The listing builds one solid part. Answer for the finished solid, in the listing's coordinates (mm). A direction names the side the tool comes from. Coordinates: 2 decimals unless noted, no trailing zeros. Order: outer loops, then holes, each group sorted by start corner. A loop starts at its lowest first (then second) coordinate and runs counter-clockwise, first axis right, second up. Notation, with made-up numbers: (-34.5, 14) -> (20.5, 14) arc R23 ccw to (20.5, 26) -> close; hole circle Ø10 at (32, 3). An arc over 180 degrees is marked (long way). Write item = value, one per line.
from build123d import *

# Parameters (mm, degrees)
SKETCH1_W           = 120
SKETCH1_H           = 120
BOSS_EXTRUDE1_DEPTH = 17
SHELL1_T            = -3
SKETCH2_W           = 124
SKETCH2_H           = 124
SKETCH2_W_2         = 120
SKETCH2_H_2         = 120
BOSS_EXTRUDE2_DEPTH = 5
SKETCH4_R           = 4.02
BOSS_EXTRUDE3_DEPTH = 14
SKETCH3_R           = 4.02
CUT_EXTRUDE1_DEPTH  = 3
FILLET1_R           = 10
SKETCH9_R           = 9.39878502
SKETCH9_R_2         = 4.690586007
SKETCH9_W           = 4.6868
SKETCH9_H           = 21.8714
BOSS_EXTRUDE7_DEPTH = 1


with BuildPart() as part:
    # Sketch1 → Boss-Extrude1 (new body)
    with BuildSketch(Plane(origin=(0, 0, 0), x_dir=(1, 0, 0), z_dir=(0, 1, 0))):
        Rectangle(SKETCH1_W, SKETCH1_H)
    extrude(amount=BOSS_EXTRUDE1_DEPTH)

    # Shell1
    shell1_openings = [part.faces().sort_by_distance(p)[0] for p in [
        (0, 0, 0),
    ]]
    offset(amount=SHELL1_T, openings=shell1_openings, kind=Kind.INTERSECTION)

    # Sketch2 → Boss-Extrude2 (add)
    with BuildSketch(Plane.XZ):
        Rectangle(SKETCH2_W, SKETCH2_H)
        Rectangle(SKETCH2_W_2, SKETCH2_H_2, mode=Mode.SUBTRACT)
    extrude(amount=-BOSS_EXTRUDE2_DEPTH)

    # Sketch4 → Boss-Extrude3 (add)
    # profile 1 of 4: a face of its own
    with BuildSketch(Plane.XZ.offset(-14)):
        with BuildLine():
            Line((-57, 42.98), (-57, 57))
            Line((-57, 57), (-42.98, 57))
            ThreePointArc((-42.98, 57), (-44.394213562, 56.414213562), (-44.98, 55))
            Line((-44.98, 55), (-44.98, 52))
            ThreePointArc((-44.98, 52), (-47.036110396, 47.036110396), (-52, 44.98))
            Line((-52, 44.98), (-55, 44.98))
            ThreePointArc((-55, 44.98), (-56.414213562, 44.394213562), (-57, 42.98))
        make_face()
        with Locations(Location((-52, 52, 0), (0, 0, 270))):
            Circle(SKETCH4_R, mode=Mode.SUBTRACT)
    # profile 2 of 4: a face of its own
    with BuildSketch(Plane.XZ.offset(-14)):
        with BuildLine():
            Line((57, 42.98), (57, 57))
            Line((57, 57), (42.98, 57))
            ThreePointArc((42.98, 57), (44.394213562, 56.414213562), (44.98, 55))
            Line((44.98, 55), (44.98, 52))
            ThreePointArc((44.98, 52), (47.036110396, 47.036110396), (52, 44.98))
            Line((52, 44.98), (55, 44.98))
            ThreePointArc((55, 44.98), (56.414213562, 44.394213562), (57, 42.98))
        make_face()
        with Locations(Location((52, 52, 0), (0, 0, 90))):
            Circle(SKETCH4_R, mode=Mode.SUBTRACT)
    # profile 3 of 4: a face of its own
    with BuildSketch(Plane.XZ.offset(-14)):
        with BuildLine():
            Line((55, -44.98), (52, -44.98))
            ThreePointArc((52, -44.98), (47.036110396, -47.036110396), (44.98, -52))
            Line((44.98, -52), (44.98, -55))
            ThreePointArc((44.98, -55), (44.394213562, -56.414213562), (42.98, -57))
            Line((42.98, -57), (57, -57))
            Line((57, -57), (57, -42.98))
            ThreePointArc((57, -42.98), (56.414213562, -44.394213562), (55, -44.98))
        make_face()
        with Locations(Location((52, -52, 0), (0, 0, 270))):
            Circle(SKETCH4_R, mode=Mode.SUBTRACT)
    # profile 4 of 4: a face of its own
    with BuildSketch(Plane.XZ.offset(-14)):
        with BuildLine():
            Line((-57, -42.98), (-57, -57))
            Line((-57, -57), (-42.98, -57))
            ThreePointArc((-42.98, -57), (-44.394213562, -56.414213562), (-44.98, -55))
            Line((-44.98, -55), (-44.98, -52))
            ThreePointArc((-44.98, -52), (-47.036110396, -47.036110396), (-52, -44.98))
            Line((-52, -44.98), (-55, -44.98))
            ThreePointArc((-55, -44.98), (-56.414213562, -44.394213562), (-57, -42.98))
        make_face()
        with Locations(Location((-52, -52, 0), (0, 0, 90))):
            Circle(SKETCH4_R, mode=Mode.SUBTRACT)
    extrude(amount=BOSS_EXTRUDE3_DEPTH)

    # Sketch3 → Cut-Extrude1 (cut)
    with BuildSketch(Plane(origin=(0, 17, 0), x_dir=(1, 0, 0), z_dir=(0, 1, 0))):
        with Locations(Location((-52, 52, 0), (0, 0, 270))):
            Circle(SKETCH3_R)
        with Locations(Location((52, 52, 0), (0, 0, 90))):
            Circle(SKETCH3_R)
        with Locations(Location((52, -52, 0), (0, 0, 270))):
            Circle(SKETCH3_R)
        with Locations(Location((-52, -52, 0), (0, 0, 90))):
            Circle(SKETCH3_R)
    extrude(amount=-CUT_EXTRUDE1_DEPTH, mode=Mode.SUBTRACT)

    # Fillet1
    fillet1_edges = [part.edges().sort_by_distance(p)[0] for p in [
        (62, 2.5, -62),
        (-62, 2.5, -62),
        (-62, 2.5, 62),
        (62, 2.5, 62),
        (60, 11, 60),
        (-60, 11, 60),
        (-60, 11, -60),
        (60, 11, -60),
    ]]
    fillet(fillet1_edges, radius=FILLET1_R)

    # Sketch9 → Boss-Extrude7 (add)
    # profile 1 of 8: a face of its own
    with BuildSketch(Plane(origin=(0, 17, 0), x_dir=(1, 0, 0), z_dir=(0, 1, 0))):
        with Locations(Location((0, 12.032739488, 0), (0, 0, 270))):
            Circle(SKETCH9_R)
        with Locations(Location((0, 12.032739488, 0), (0, 0, 270))):
            Circle(SKETCH9_R_2, mode=Mode.SUBTRACT)
    # profile 2 of 8: a face of its own
    with BuildSketch(Plane(origin=(0, 17, 0), x_dir=(1, 0, 0), z_dir=(0, 1, 0))):
        with BuildLine():
            Line((-13.44305, 20.375947386), (-17.50480026, 22.896805886))
            ThreePointArc((-17.50480026, 22.896805886), (0.002640651, 32.634825883), (17.507584665, 22.892318209))
            Line((17.507584665, 22.892318209), (13.445188322, 20.372501014))
            ThreePointArc((13.445188322, 20.372501014), (0.002027924, 27.854392601), (-13.44305, 20.375947386))
        make_face()
    # profile 3 of 8: a face of its own
    with BuildSketch(Plane(origin=(0, 17, 0), x_dir=(1, 0, 0), z_dir=(0, 1, 0))):
        with BuildLine():
            Line((-40.2286, -27.927144715), (-40.2286, 3.597555285))
            ThreePointArc((-40.2286, 3.597555285), (-37.592561031, 9.961516315), (-31.2286, 12.597555285))
            Line((-31.2286, 12.597555285), (-14.988446655, 12.597555285))
            Line((-14.988446655, 12.597555285), (-14.988446655, 7.597555285))
            Line((-14.988446655, 7.597555285), (-31.2286, 7.597555285))
            ThreePointArc((-31.2286, 7.597555285), (-34.057027125, 6.42598241), (-35.2286, 3.597555285))
            Line((-35.2286, 3.597555285), (-35.2286, -27.927144715))
            ThreePointArc((-35.2286, -27.927144715), (-34.057027125, -30.75557184), (-31.2286, -31.927144715))
            Line((-31.2286, -31.927144715), (31.2286, -31.927144715))
            ThreePointArc((31.2286, -31.927144715), (34.057027125, -30.75557184), (35.2286, -27.927144715))
            Line((35.2286, -27.927144715), (35.2286, 3.597555285))
            ThreePointArc((35.2286, 3.597555285), (34.057027125, 6.42598241), (31.2286, 7.597555285))
            Line((31.2286, 7.597555285), (14.988446655, 7.597555285))
            Line((14.988446655, 7.597555285), (14.988446655, 12.597555285))
            Line((14.988446655, 12.597555285), (31.2286, 12.597555285))
            ThreePointArc((31.2286, 12.597555285), (37.592561031, 9.961516315), (40.2286, 3.597555285))
            Line((40.2286, 3.597555285), (40.2286, -27.927144715))
            ThreePointArc((40.2286, -27.927144715), (37.592561031, -34.291105746), (31.2286, -36.927144715))
            Line((31.2286, -36.927144715), (-31.2286, -36.927144715))
            ThreePointArc((-31.2286, -36.927144715), (-37.592561031, -34.291105746), (-40.2286, -27.927144715))
        make_face()
    # profile 4 of 8: a face of its own
    with BuildSketch(Plane(origin=(0, 17, 0), x_dir=(1, 0, 0), z_dir=(0, 1, 0))):
        with BuildLine():
            Line((-22.967626314, 26.287219035), (-26.8861, 28.719155285))
            ThreePointArc((-26.8861, 28.719155285), (0.004055848, 43.676045714), (26.890376645, 28.712262541))
            Line((26.890376645, 28.712262541), (22.971279665, 26.281330863))
            ThreePointArc((22.971279665, 26.281330863), (0.003464735, 39.064240253), (-22.967626314, 26.287219035))
        make_face()
    # profile 5 of 8: a face of its own
    with BuildSketch(Plane(origin=(0, 17, 0), x_dir=(1, 0, 0), z_dir=(0, 1, 0))):
        with BuildLine():
            Line((-27.8078, -24.037744715), (-27.8077, -2.166344715))
            Line((-27.8077, -2.166344715), (-19.6684, -2.322544715))
            ThreePointArc((-19.6684, -2.322544715), (-14.083780395, -7.46632893), (-16.7627, -14.570544715))
            Line((-16.7627, -14.570544715), (-13.694775607, -23.959644715))
            Line((-13.694775607, -23.959644715), (-18.653, -23.959644715))
            Line((-18.653, -23.959644715), (-21.3088, -15.757844715))
            Line((-21.3088, -15.757844715), (-23.121, -15.757844715))
            Line((-23.121, -15.757844715), (-23.121, -24.037744715))
            Line((-23.121, -24.037744715), (-27.8078, -24.037744715))
        make_face()
        with BuildLine():
            Line((-23.1211, -6.853044715), (-23.1211, -11.071144715))
            Line((-23.1211, -11.071144715), (-20.688080887, -11.071144715))
            ThreePointArc((-20.688080887, -11.071144715), (-18.579030887, -8.962094715), (-20.688080887, -6.853044715))
            Line((-20.688080887, -6.853044715), (-23.1211, -6.853044715))
        make_face(mode=Mode.SUBTRACT)
    # profile 6 of 8: a face of its own
    with BuildSketch(Plane(origin=(0, 17, 0), x_dir=(1, 0, 0), z_dir=(0, 1, 0))):
        Polygon((-9.5295, -2.166244715), (-9.5295, -24.037744715), (-4.8428, -24.037744715), (-4.8428, -15.289144715), (-0.781, -15.289144715), (-0.781, -10.602344715), (-4.8428, -10.602344715), (-4.8428, -6.853044715), (1.25, -6.853044715), (1.25, -2.166244715), align=None)
    # profile 7 of 8: a face of its own
    with BuildSketch(Plane(origin=(0, 17, 0), x_dir=(1, 0, 0), z_dir=(0, 1, 0))):
        with Locations((7.4989, -13.102044715)):
            Rectangle(SKETCH9_W, SKETCH9_H)
    # profile 8 of 8: a face of its own
    with BuildSketch(Plane(origin=(0, 17, 0), x_dir=(1, 0, 0), z_dir=(0, 1, 0))):
        with BuildLine():
            Line((13.904, -2.135144715), (13.904, -24.068944715))
            Line((13.904, -24.068944715), (22.62153415, -24.068944715))
            ThreePointArc((22.62153415, -24.068944715), (29.187351473, -13.102044715), (22.62153415, -2.135144715))
            Line((22.62153415, -2.135144715), (13.904, -2.135144715))
        make_face()
        with BuildLine():
            Line((18.5908, -6.806144715), (18.5908, -19.351044715))
            Line((18.5908, -19.351044715), (20.808626637, -19.351044715))
            ThreePointArc((20.808626637, -19.351044715), (25.011270759, -13.078594715), (20.808626637, -6.806144715))
            Line((20.808626637, -6.806144715), (18.5908, -6.806144715))
        make_face(mode=Mode.SUBTRACT)
    extrude(amount=BOSS_EXTRUDE7_DEPTH)


solid = part.part
Q1. The mould has two halves that part along X. Classify faces 1 (the face through (-53, 7, -44.98)), 2 (the face through (-21, 18, 13)), 3 (the face through (37.522, 17.493, -10.031)): released by +X, released by -X, zero draft, split by the parting line, or undercut.
The answers:
face_1 = undercut
face_2 = zero draft
face_3 = released by +X
Q2. Section B-B, the plane x = -46.5 is taken. Give the vertices of the cut face in (y, z), plus the area to 3 significant figures.
The answers:
outline = (0, -62) -> (5, -62) -> (5, -60) -> (17, -60) -> (17, 60) -> (5, 60) -> (5, 62) -> (0, 62) -> (0, 47.64) -> (14, 47.64) -> (14, -47.64) -> (0, -47.64) -> close
area = 726 mm2
Q3. A tool of negligible diameter and unlimited length cuts with its end or side. For faces 4 (the face through (-56.99, 11.08, -57.15)), 5 (the face through (60, 11, 1)), 6 (the face through (-1, 11, -60)), 7 (the face through (-56.99, 11.08, 57.15)), 8 (the face through (0.227, 17.493, -27.853)), from which of +Z, -Z, +X, -X, +Y, -Y can it reach the whole face along a straight path? Write none if from no direction.
The answers:
face_4 = -Z, -X, +Y
face_5 = +Z, -Z, +X, +Y
face_6 = -Z, +X, -X, +Y
face_7 = +Z, -X, +Y
face_8 = +Y
Q4. Each of these flat-tipped pins is pushed along its axis until it touches: pin 1 Ø1 at (x, y) = (-18, 10.5) entering from -Z; pin 2 Ø3 at (x, z) = (21.5, 11.5) entering from +Y; pin 3 Ø1.5 at (y, z) = (15, 37) entering from -X; pin 4 Ø7 at (y, z) = (7, 21.5) entering from -X. Where does it stop, or does it pass through?
The answers:
pin_1 = -60
pin_2 = 17
pin_3 = -60
pin_4 = -62
Q5. Find the intervals of material crossed by line 1 along X through (y, z) = (3, 52); line 2 along X through (y, z) = (10.25, 9.5), in increasing order.
The answers:
line_1 = -62 to -56.02, -47.98 to -44.98, 44.98 to 47.98, 56.02 to 62
line_2 = -60 to -57, 57 to 60
